The listing builds one solid part. Answer for the finished solid, in the listing's coordinates (mm). Face numbers are marked on the shaded views. Give positions to 0.01 mm unless a question says otherwise; leave off trailing zeros. Write each loop counter-clockwise with the first axis right and the second up, starting at its lowest first coordinate (ties: lowest second). Pieces come first, ordered by that corner, then holes. Notation, with made-up numbers: M -2,-26 L 11,-26 A27 cw 11,-5 Z; hole C -26,-38 d1. An arc over 180 degrees is marked long. Return JSON: item names as keys, results as strings.
from build123d import *

# Parameters (mm, degrees)
ESBO_O1_W                = 34
ESBO_O1_H                = 34
RESSALTO_EXTRUS_O1_DEPTH = 2.5
ESBO_O2_R                = 7.5
ESBO_O2_R_2              = 4
CORTE_EXTRUS_O1_DEPTH    = 1
ESBO_O3_R                = 1.25
CORTE_EXTRUS_O2_DEPTH    = 5
ESBO_O4_R                = 1
CORTE_EXTRUS_O3_DEPTH    = 10


with BuildPart() as part:
    # Esboço1 → Ressalto-extrusão1 (new, symmetric)
    with BuildSketch(Plane.XY):
        Rectangle(ESBO_O1_W, ESBO_O1_H)
    extrude(amount=RESSALTO_EXTRUS_O1_DEPTH, both=True)

    # Esboço2 → Corte-extrusão1 (cut)
    with BuildSketch(Plane.XY.offset(2.5)):
        Circle(ESBO_O2_R)
        Circle(ESBO_O2_R_2, mode=Mode.SUBTRACT)
    extrude(amount=-CORTE_EXTRUS_O1_DEPTH, mode=Mode.SUBTRACT)

    # Esboço3 → Corte-extrusão2 (cut)
    with BuildSketch(Plane.XY.offset(2.5)):
        Circle(ESBO_O3_R)
    extrude(amount=-CORTE_EXTRUS_O2_DEPTH, mode=Mode.SUBTRACT)

    # Esboço4 → Corte-extrusão3 (cut)
    with BuildSketch(Plane.ZY.offset(17)):
        with Locations((0, 11)):
            Circle(ESBO_O4_R)
        with Locations((0, -11)):
            Circle(ESBO_O4_R)
    corte_extrus_o3 = extrude(amount=-CORTE_EXTRUS_O3_DEPTH, mode=Mode.SUBTRACT)

    # Espelhar1: Corte-extrusão3 across plane
    add(corte_extrus_o3.mirror(Plane(origin=(0, 0, 0), x_dir=(0, 0, 1), z_dir=(1, 0, 0))), mode=Mode.SUBTRACT)


solid = part.part
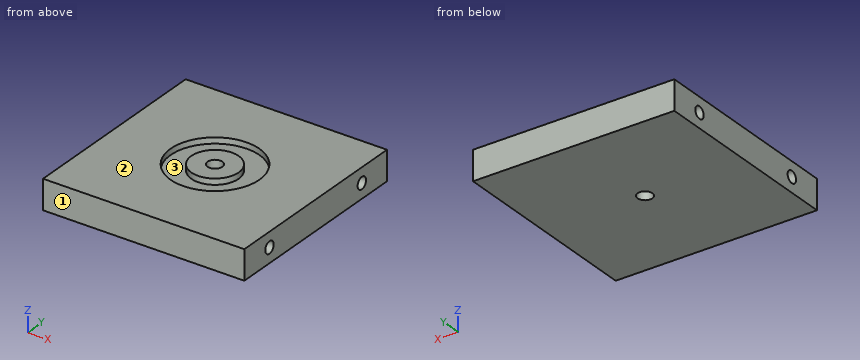
Item 1: A cutting plane is placed at C-C, the plane z = 0. Write down the section's boundary in (x, y), plus the area to 3 significant figures.
Geometry results:
{"outline": "M -17,-17 L 17,-17 L 17,-12 L 7,-12 L 7,-10 L 17,-10 L 17,10 L 7,10 L 7,12 L 17,12 L 17,17 L -17,17 L -17,12 L -7,12 L -7,10 L -17,10 L -17,-10 L -7,-10 L -7,-12 L -17,-12 Z; hole C 0,0 d2.5", "area": "1,070 mm2"}
Item 2: A cutting plane is placed at A-A, the plane z = 2. Write down the section's boundary in (x, y).
Geometry results:
{"outline": "M -17,-17 L 17,-17 L 17,17 L -17,17 Z; C 0,0 d8; hole C 0,0 d15; hole C 0,0 d2.5"}
Item 3: Given pin 1 Ø1.6 at (y, z) = (-11, 0) entering from +X; pin 2 Ø2.5 at (y, z) = (-11, 0) entering from -X, each flat-ended and moving along its own axis, determine where each tip first touches the part or whether it passes through.
Geometry results:
{"pin 1": "stops at x = 7", "pin 2": "stops at x = -17"}
Item 4: Find the intervals of material crossed by line 1 (Y direction, x = -9.5, z = 0); line 2 (Y direction, x = 0, z = 2.1); line 3 (Y direction, x = 0, z = 1.05), in increasing order.
Geometry results:
{"line 1": "y = -17 to -12, -10 to 10, 12 to 17", "line 2": "y = -17 to -7.5, -4 to -1.25, 1.25 to 4, 7.5 to 17", "line 3": "y = -17 to -1.25, 1.25 to 17"}
Item 5: A cutting plane is placed at D-D, the plane x = 8. Write down the section's boundary in (y, z).
Geometry results:
{"outline": "M -17,-2.5 L 17,-2.5 L 17,2.5 L -17,2.5 Z; hole C -11,0 d2; hole C 11,0 d2"}
Item 6: Determine the mould class of the marked faces 1, 2 and 3 for opening direction Y: +Y half, -Y half, draft (parallel to the pull), parting line (faces both ways), or undercut.
Geometry results:
{"face 1": "-Y half", "face 2": "draft", "face 3": "undercut"}
Item 7: A cutting plane is placed at B-B, the plane y = 11. Write down the section's boundary in (x, z).
Geometry results:
{"outline": "M -17,-2.5 L 17,-2.5 L 17,-1 L 7,-1 L 7,1 L 17,1 L 17,2.5 L -17,2.5 L -17,1 L -7,1 L -7,-1 L -17,-1 Z"}
